The figure shows three views and two pictorial views of one solid part (mm, origin at its lowest corner). Answer the questions. A direction names the side the tool comes from. Round coordinates to 2 decimals unless told otherwise and drop trailing zeros. Order: outer loops, then holes, each group sorted by start corner. A loop starts at its lowest first (then second) coordinate and runs counter-clockwise, first axis right, second up. Notation, with made-up numbers: (-37.75, 40) - (-5.75, 40) arc R13 ccw to (-5.75, 59) - close; hole circle Ø1 at (-18, 21). An arc over 180 degrees is marked (long way). Write item = value, one per line.
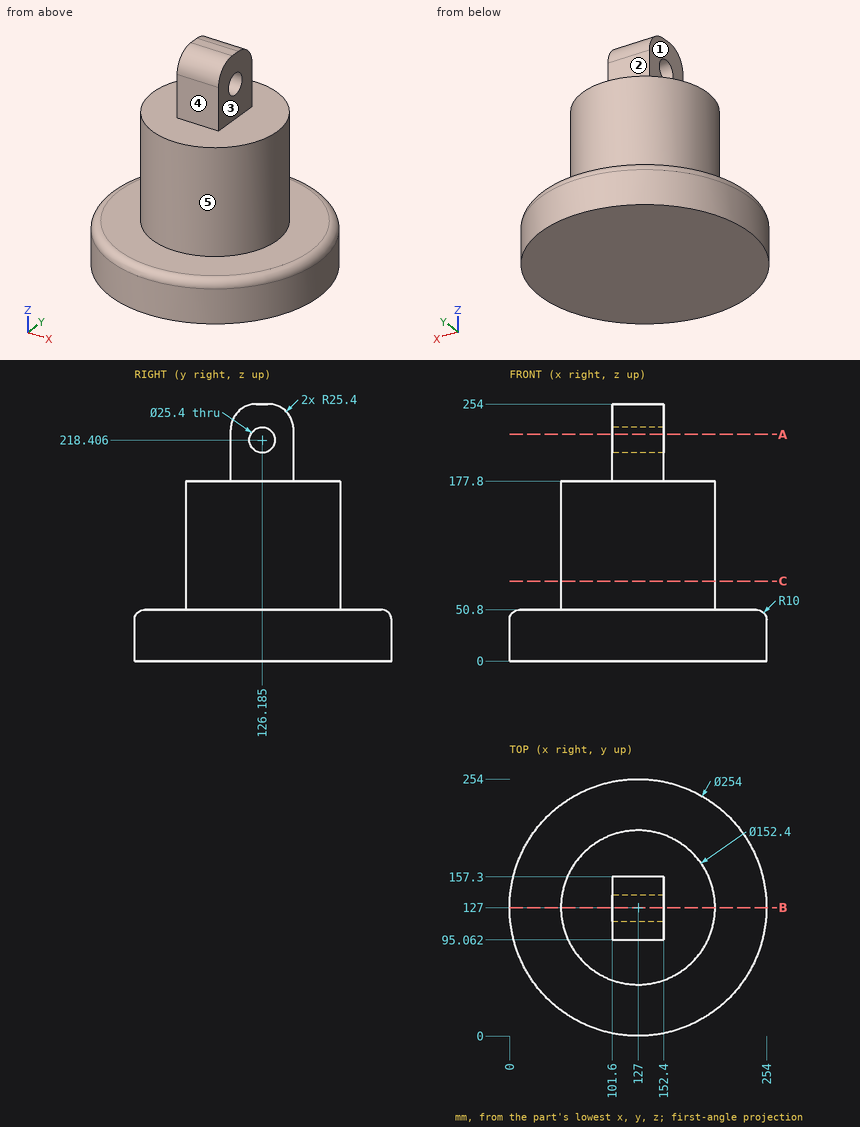
Q1. Section C-C on z = 79 is taken. Determine the outline of the cut face in (x, y).
Model answer:
outline = circle Ø152.4 at (127, 127)
Q2. Flat-ended cylindrical pins translate along their axes: P1, Ø18.5, axis at y = 131.5, z = 229, coming from the +X side; P2, Ø18.5, axis at y = 115, z = 229.5, coming from the -X side; P3, Ø8, axis at x = 163.5, y = 62, coming from the +Z side. Find the tip coordinate at first contact, or state that the pin passes through.
Model answer:
P1 = 152.4
P2 = 101.6
P3 = 177.8
Q3. Find the intervals of material crossed by line 1 (Z direction, x = 13, y = 158) (1 decimal); line 2 (Z direction, x = 42, y = 192); line 3 (Z direction, x = 121.5, y = 131.5), in increasing order. Write a range as from..to.
Model answer:
line_1 = 0..50.7
line_2 = 0..50.8
line_3 = 0..206.87, 229.94..254
Q4. Section B-B on y = 127 is taken. Determine the outline of the cut face in (x, z), then the cut area to 3 significant figures.
Model answer:
outline = (0, 0) - (254, 0) - (254, 40.8) arc R10 ccw to (244, 50.8) - (203.2, 50.8) - (203.2, 177.8) - (152.4, 177.8) - (152.4, 205.73) - (101.6, 205.73) - (101.6, 177.8) - (50.8, 177.8) - (50.8, 50.8) - (10, 50.8) arc R10 ccw to (0, 40.8) - close; (101.6, 231.08) - (152.4, 231.08) - (152.4, 254) - (101.6, 254) - close
area = 34,800 mm^2
Q5. Section A-A on z = 224 is taken. Determine the outline of the cut face in (x, y).
Model answer:
outline = (101.6, 95.06) - (152.4, 95.06) - (152.4, 114.78) - (101.6, 114.78) - close; (101.6, 137.59) - (152.4, 137.59) - (152.4, 157.3) - (101.6, 157.3) - close
Q6. For the marked faces 1, 2, 3, 4 and 5, determine the directions among +Z, -Z, +X, -X, +Y, -Y from which every point of the face is accessible in a straight line to the end or side of a thin tool.
Model answer:
face_1 = +Z, -X, +Y, -Y
face_2 = +Z, +X, -X, +Y
face_3 = +Z, +X, +Y, -Y
face_4 = +Z, +X, -X, -Y
face_5 = +Z
